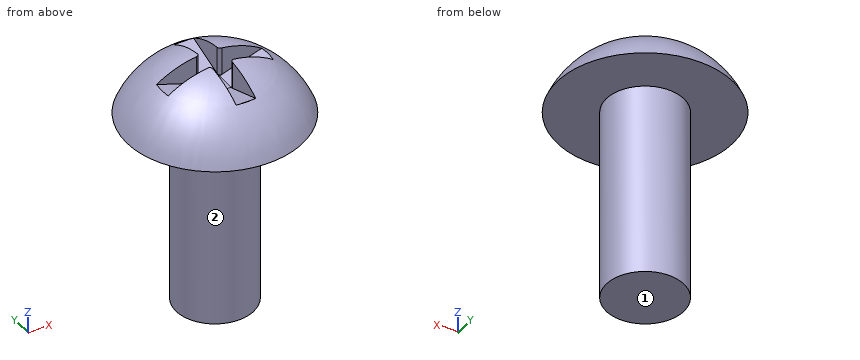
from build123d import *

# Parameters (mm, degrees)
F3_R           = 2
F4_DEPTH       = 10
F5_W           = 1
F5_H           = 0.8
F6_DEPTH       = 3
F6_DEPTH_BACK  = 3
F7_W           = 1
F7_H           = 0.8
F8_DEPTH       = 3
F8_DEPTH_BACK  = 3
F10_DEPTH      = 0.5
F10_DEPTH_BACK = 0.5
F11_T4_DEPTH   = 1
F12_T1_DEPTH   = 1
F13_T4_DEPTH   = 2.2322667456
F13_T10_DEPTH  = 1.8596499945
F13_T16_DEPTH  = 2.2322667452
F13_T22_DEPTH  = 1.859649995


# Not quite as in the source:
# - a fillet or chamfer that OpenCascade refuses, or shapes differently, is made with other operations: its cross-section is extruded or revolved along the edge and cut away or added


with BuildPart() as f2:
    # F0 (on Front) → F2 (revolve)
    with BuildSketch(Plane.XZ):
        with BuildLine():
            Line((0, 0), (0, 2.9999249461))
            ThreePointArc((0, 2.9999249461), (-2.7199502547, 2.1887322683), (-4.5270512497, 0))
            Line((-4.5270512497, 0), (0, 0))
        make_face()
    revolve(axis=Axis((0, 0, 1.5515517443), (0, 0, -1)))

    # F3 (on face) → F4 (join)
    with BuildSketch(Plane(origin=(0, 0, 0), x_dir=(1, 0, 0), z_dir=(0, 0, -1))):
        Circle(F3_R)
    extrude(amount=F4_DEPTH)

    # F5 (on Front) → F6 (cut, two sides)
    with BuildSketch(Plane.XZ) as f6_sk:
        with Locations((0, 2.6000668348)):
            Rectangle(F5_W, F5_H)
    extrude(amount=-F6_DEPTH, mode=Mode.SUBTRACT)
    extrude(f6_sk.sketch, amount=F6_DEPTH_BACK, mode=Mode.SUBTRACT)

    # F7 (on Right) → F8 (cut, two sides)
    with BuildSketch(Plane.YZ) as f8_sk:
        with Locations((0, 2.5815645484)):
            Rectangle(F7_W, F7_H)
    extrude(amount=F8_DEPTH, mode=Mode.SUBTRACT)
    extrude(f8_sk.sketch, amount=-F8_DEPTH_BACK, mode=Mode.SUBTRACT)

    # F9 (on Front) → F10 (cut, two sides)
    with BuildSketch(Plane.XZ) as f10_sk:
        Polygon((0.5315009621, 1.4676835854), (2.7381633418, 2.1851595957), (-2.7381633418, 2.1851595957), (-0.5315009621, 1.4676835854), (0, 1.4676835854), align=None)
    extrude(amount=F10_DEPTH, mode=Mode.SUBTRACT)
    extrude(f10_sk.sketch, amount=-F10_DEPTH_BACK, mode=Mode.SUBTRACT)

    # F11: chamfer of 0.733 x 2.18 on 1 edges, made by hand


with BuildPart() as f11_tool2:
    # F11_s3 → F11_t4 (new body)
    with BuildSketch(Plane.YZ.offset(0.5)):
        Polygon((2.68, 2.2000668348), (0.5, 1.4670668348), (0.5, 2.2000668348), align=None)
    extrude(amount=-F11_T4_DEPTH)

    split(bisect_by=Plane.XY.offset(1.4676835854), keep=Keep.TOP)


with BuildPart() as f2_1:
    add(f2.part)

    # F11_t1: cut F11_tool2
    add(f11_tool2.part, mode=Mode.SUBTRACT)

    # F12: chamfer of 2.183 x 0.73 on 1 edges, made by hand

    # F12_s2 → F12_t1 (cut)
    with BuildSketch(Plane.YZ.offset(-0.5)):
        Polygon((-0.5, 1.4700668348), (-2.683, 2.2000668348), (-0.5, 2.2000668348), align=None)
    extrude(amount=F12_T1_DEPTH, mode=Mode.SUBTRACT)

    # F13: fillet of radius 0.15 on 4 edges, made by hand


with BuildPart() as f13_tool2:
    # F13_s3 → F13_t4 (new body)
    with BuildSketch(Plane.XY.offset(3.3273335804)):
        with BuildLine():
            ThreePointArc((0.65, -0.5), (0.5439339828, -0.5439339828), (0.5, -0.65))
            Line((0.5, -0.65), (0.5, -0.5))
            Line((0.5, -0.5), (0.65, -0.5))
        make_face()
    extrude(amount=-F13_T4_DEPTH)

    split(bisect_by=Plane(origin=(-0.3807624945, 0, 1.1710694992), x_dir=(0, 1, 0), z_dir=(-0.309207193, 0, 0.950994696)), keep=Keep.TOP)

    split(bisect_by=Plane(origin=(0, 0.3918613388, 1.1718264421), x_dir=(1, 0, 0), z_dir=(0, 0.3171399402, 0.9483787526)), keep=Keep.TOP)


with BuildPart() as f2_2:
    add(f2_1.part)

    # F13_t1: cut F13_tool2
    add(f13_tool2.part, mode=Mode.SUBTRACT)


with BuildPart() as f13_tool8:
    # F13_s9 → F13_t10 (new body)
    with BuildSketch(Plane.XY.offset(3.3273335799)):
        with BuildLine():
            ThreePointArc((0.5, 0.65), (0.5439339828, 0.5439339828), (0.65, 0.5))
            Line((0.65, 0.5), (0.5, 0.5))
            Line((0.5, 0.5), (0.5, 0.65))
        make_face()
    extrude(amount=-F13_T10_DEPTH)

    split(bisect_by=Plane(origin=(0, -0.3923936318, 1.16700971), x_dir=(1, 0, 0), z_dir=(0, -0.3187050207, 0.9478539496)), keep=Keep.TOP)

    split(bisect_by=Plane(origin=(-0.3807624945, 0, 1.1710694992), x_dir=(0, 1, 0), z_dir=(-0.309207193, 0, 0.950994696)), keep=Keep.TOP)


with BuildPart() as f2_3:
    add(f2_2.part)

    # F13_t7: cut F13_tool8
    add(f13_tool8.part, mode=Mode.SUBTRACT)


with BuildPart() as f13_tool14:
    # F13_s15 → F13_t16 (new body)
    with BuildSketch(Plane.XY.offset(1.0950668348)):
        with BuildLine():
            ThreePointArc((-0.65, -0.5), (-0.5439339828, -0.5439339828), (-0.5, -0.65))
            Line((-0.5, -0.65), (-0.5, -0.5))
            Line((-0.5, -0.5), (-0.65, -0.5))
        make_face()
    extrude(amount=F13_T16_DEPTH)

    split(bisect_by=Plane(origin=(0.3807624945, 0, 1.1710694992), x_dir=(0, 1, 0), z_dir=(0.309207193, 0, 0.950994696)), keep=Keep.TOP)

    split(bisect_by=Plane(origin=(0, 0.3918613388, 1.1718264421), x_dir=(1, 0, 0), z_dir=(0, 0.3171399402, 0.9483787526)), keep=Keep.TOP)


with BuildPart() as f2_4:
    add(f2_3.part)

    # F13_t13: cut F13_tool14
    add(f13_tool14.part, mode=Mode.SUBTRACT)


with BuildPart() as f13_tool20:
    # F13_s21 → F13_t22 (new body)
    with BuildSketch(Plane.XY.offset(3.3273335804)):
        with BuildLine():
            ThreePointArc((-0.65, 0.5), (-0.5439339828, 0.5439339828), (-0.5, 0.65))
            Line((-0.5, 0.65), (-0.5, 0.5))
            Line((-0.5, 0.5), (-0.65, 0.5))
        make_face()
    extrude(amount=-F13_T22_DEPTH)

    split(bisect_by=Plane(origin=(0.3807624945, 0, 1.1710694992), x_dir=(0, 1, 0), z_dir=(0.309207193, 0, 0.950994696)), keep=Keep.TOP)

    split(bisect_by=Plane(origin=(0, -0.3923936318, 1.16700971), x_dir=(1, 0, 0), z_dir=(0, -0.3187050207, 0.9478539496)), keep=Keep.TOP)


with BuildPart() as f2_5:
    add(f2_4.part)

    # F13_t19: cut F13_tool20
    add(f13_tool20.part, mode=Mode.SUBTRACT)


solid = f2_5.part
Part model, mm, in its own coordinate system. Face numbers are marked on the shaded views. A direction names the side the tool comes from. Coordinates: 2 decimals unless noted, no trailing zeros. Loops run counter-clockwise (first coordinate to the right, second up) from the corner with the lowest first, then second, coordinate; pieces in that order, holes last. Notation, with made-up numbers: (-20.75, 23) -> (-9.75, 23) arc R13 ccw to (-9.75, 37) -> close; hole circle Ø5 at (38.25, 73). An arc over 180 degrees is marked (long way). Use a Markdown table: item, result. Add a question column.
Item 1: Band-saw the part on A-A on z = -1.5. Write the cut outline in (x, y), plus the area to 3 significant figures.
Item 2: Flat gauge pins, fed straight in: P1, Ø5, axis at x = 1.5, z = -8.5, coming from the -Y side; P2, Ø2, axis at y = -0.5, z = 0, coming from the +X side; P3, Ø1.6, axis at x = -1.5, z = 2.5, coming from the +Y side; P4, Ø1.1, axis at y = -2, z = 2.5, coming from the -X side. Where does each tip first touch, or does it go through?
Item 3: Probe probe 1 along Y at (x, z) = (0, -1.75); probe 2 along X at (y, z) = (1, -6); probe 3 along X at (y, z) = (-1.75, -3.75). List the from-to ranges inside material, lowest first.
Item 4: Which spindle directions (+Z, -Z, +X, -X, +Y, -Y) get a long thin tool onto all of the face, cutting with end or side? Do the marked faces 1 and 2. Say none if no direction does.
Geometry says:
| question | item | result |
|---|---|---|
| 1 | outline | circle Ø4 at (0, 0) |
| 1 | area | 12.6 mm² |
| 2 | P1 | y = -2 |
| 2 | P2 | x = 4.53 |
| 2 | P3 | y = 3.05 |
| 2 | P4 | x = -2.4 |
| 3 | probe 1 | -2 to 2 |
| 3 | probe 2 | -1.73 to 1.73 |
| 3 | probe 3 | -0.97 to 0.97 |
| 4 | face 1 | -Z, +X, -X, +Y, -Y |
| 4 | face 2 | -Z |
